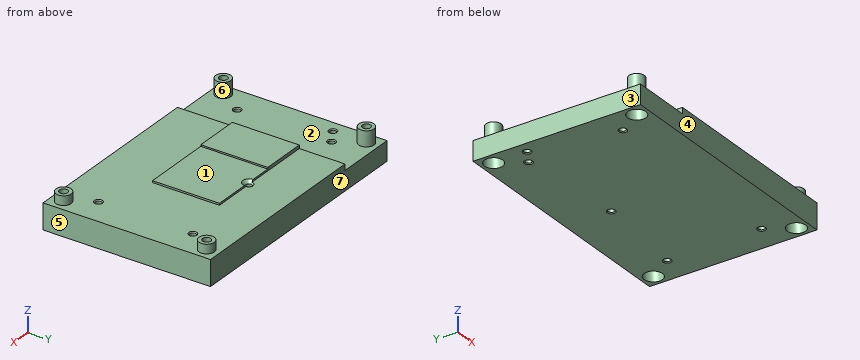
```python
from build123d import *

# Parameters (mm, degrees)
SKETCH1_W                               = 84
SKETCH1_H                               = 55
EXTRUDE1_DEPTH                          = 11.4
F_2_7_2_7_DIAMETER_HOLE1_D              = 2.7
SKETCH6_OUTSIDE_W                       = 106.21
SKETCH6_OUTSIDE_H                       = 77.21
SKETCH6_OUTSIDE_R                       = 2.5
EXTRUDE2_DEPTH                          = 3
SKETCH7_W                               = 15
SKETCH7_H                               = 22
EXTRUDE3_DEPTH                          = 1.1
SKETCH8_W                               = 26.471562954
SKETCH8_H                               = 62.575334395
SKETCH8_R                               = 2.5
EXTRUDE6_DEPTH                          = 2
SKETCH9_W                               = 23
SKETCH9_H                               = 22
EXTRUDE7_DEPTH                          = 0.6
M2_5X0_45_TAPPED_HOLE1_D                = 2.05
CBORE_FOR_M5_HEX_HEAD_BOLT1_D           = 2.7
CBORE_FOR_M5_HEX_HEAD_BOLT1_CBORE_D     = 6
CBORE_FOR_M5_HEX_HEAD_BOLT1_CBORE_DEPTH = 3.5
CHAMFER1_SIZE                           = 0.3


with BuildPart() as part:
    # Sketch1 → Extrude1 (new body)
    with BuildSketch(Plane.XY):
        Rectangle(SKETCH1_W, SKETCH1_H)
    extrude(amount=EXTRUDE1_DEPTH)

    # 2.7 _2.7_ Diameter Hole1 (through all)
    with Locations(Plane.XY.offset(11.4)):
        with Locations((-38, 23.5), (38, 23.5), (38, -23.5), (-38, -23.5)):
            Hole(F_2_7_2_7_DIAMETER_HOLE1_D / 2)

    # Sketch6 outside → Extrude2 (cut)
    with BuildSketch(Plane.XY.offset(11.4)):
        Rectangle(SKETCH6_OUTSIDE_W, SKETCH6_OUTSIDE_H)
        with Locations((-38, 23.5)):
            Circle(SKETCH6_OUTSIDE_R, mode=Mode.SUBTRACT)
        with Locations((-38, -23.5)):
            Circle(SKETCH6_OUTSIDE_R, mode=Mode.SUBTRACT)
        with Locations((38, 23.5)):
            Circle(SKETCH6_OUTSIDE_R, mode=Mode.SUBTRACT)
        with Locations((38, -23.5)):
            Circle(SKETCH6_OUTSIDE_R, mode=Mode.SUBTRACT)
    extrude(amount=-EXTRUDE2_DEPTH, mode=Mode.SUBTRACT)

    # Sketch7 → Extrude3 (add)
    with BuildSketch(Plane.XY.offset(8.4)):
        with Locations((-14.5, 1.5)):
            Rectangle(SKETCH7_W, SKETCH7_H)
    extrude(amount=EXTRUDE3_DEPTH)

    # Sketch8 → Extrude6 (cut)
    with BuildSketch(Plane.XY.offset(8.4)):
        with Locations((-35.235781477, -1.105270853)):
            Rectangle(SKETCH8_W, SKETCH8_H)
        with Locations((-38, -23.5)):
            Circle(SKETCH8_R, mode=Mode.SUBTRACT)
        with Locations((-38, 23.5)):
            Circle(SKETCH8_R, mode=Mode.SUBTRACT)
    extrude(amount=-EXTRUDE6_DEPTH, mode=Mode.SUBTRACT)

    # Sketch9 → Extrude7 (add)
    with BuildSketch(Plane.XY.offset(8.4)):
        with Locations((4.5, 1.5)):
            Rectangle(SKETCH9_W, SKETCH9_H)
    extrude(amount=EXTRUDE7_DEPTH)

    # M2.5x0.45 Tapped Hole1 (through all)
    with Locations(Plane.XY.offset(11.4)):
        with Locations((-33, 15.5), (33, 15.5), (33, -15.5), (-33, -15.5), (2, 12.5), (-38, 12.5)):
            Hole(M2_5X0_45_TAPPED_HOLE1_D / 2)

    # CBORE for M5 Hex Head Bolt1 (through all)
    with Locations(Plane(origin=(0, 0, 0), x_dir=(-1, 0, 0), z_dir=(0, 0, -1))):
        with Locations((-38, 23.5), (-38, -23.5), (38, 23.5), (38, -23.5)):
            CounterBoreHole(CBORE_FOR_M5_HEX_HEAD_BOLT1_D / 2, CBORE_FOR_M5_HEX_HEAD_BOLT1_CBORE_D / 2, CBORE_FOR_M5_HEX_HEAD_BOLT1_CBORE_DEPTH)

    # Chamfer1
    chamfer1_edges = [part.edges().sort_by_distance(p)[0] for p in [
        (-36.975, 12.5, 0),
        (-36.975, 12.5, 6.4),
        (3.025, 12.5, 0),
        (-31.975, -15.5, 0),
        (-31.975, -15.5, 6.4),
        (34.025, -15.5, 8.4),
        (34.025, -15.5, 0),
        (34.025, 15.5, 8.4),
        (34.025, 15.5, 0),
        (-31.975, 15.5, 0),
        (-31.975, 15.5, 6.4),
    ]]
    chamfer(chamfer1_edges, length=CHAMFER1_SIZE)

    # Sketch12 → Cut-Revolve1 (revolve, cut)
    with BuildSketch(Plane.ZY.offset(-2), mode=Mode.PRIVATE) as cut_revolve1_sk:
        Polygon((6.996424716, 12.489411428), (9.321943828, 14.81493054), (9.321943828, 12.489411428), align=None)
    revolve(cut_revolve1_sk.sketch.rotate(Axis((2, 12.489411428, 7.765521671), (0, 0, 1)), 270.302801858), axis=Axis((2, 12.489411428, 7.765521671), (0, 0, 1)), mode=Mode.SUBTRACT)  # turned: the seam where the file's is


solid = part.part
```
CAD build for the part. Positions are in the model's coordinates, mm. Face numbers are marked on the shaded views. A direction names the side the tool comes from. Round coordinates to 2 decimals unless told otherwise and drop trailing zeros. Write each loop counter-clockwise with the first axis right and the second up, starting at its lowest first coordinate (ties: lowest second). Pieces come first, ordered by that corner, then holes. Notation, with made-up numbers: (42.5, -10) - (63.5, -10) arc R12 ccw to (63.5, 5) - close; hole circle Ø9 at (53, -2.5). An arc over 180 degrees is marked (long way). Return JSON: item names as keys, results as strings. Group by question number.
Item 1: 3-axis set-ups, long thin cutter, end or side, ignore diameter. For the marked faces 1, 2 and 3: which of +Z, -Z, +X, -X, +Y, -Y reach the whole face in a straight line?
Item 2: Band-saw the part on A-A on x = 38. List the corners of the cut face in (y, z), plus the area to 3 significant figures.
Item 3: Band-saw the part on B-B on z = 2. State how many separate pieces and enclosed holes the cut face has, plus the area to 3 significant figures.
Item 4: Probe probe 1 along Y at (x, z) = (-38, 7.5); probe 2 along Y at (x, z) = (-33, 3.7) (3 decimals); probe 3 along Y at (x, z) = (-38, 3.45) (3 decimals). List the from-to ranges inside material, lowest first.
Item 5: Mould opens along Y. For the marked faces 4, 5, 6 and 7 say: +Y half, -Y half, draft (parallel to the pull), parting line (faces both ways), or undercut.
Item 6: Band-saw the part on D-D on x = -8. List the corners of the cut face in (y, z).
Item 7: Band-saw the part on C-C on y = -15.5. List the corners of the cut face in (x, z) (3 decimals), plus the area to 3 significant figures.
Item 8: Flat gauge pins, fed straight in: pin 1 Ø3.5 at (x, y) = (2, 12.5) entering from +Z; pin 2 Ø2.5 at (y, z) = (-5.5, 8) entering from -X; pin 3 Ø16 at (x, y) = (-28, -11.5) entering from +Z. Where does each tip first touch, or does it go through?
Resolved:
{
 "1": {"face 1": "+Z, +X, +Y, -Y", "face 2": "+Z", "face 3": "+Z, -Z, -X, +Y, -Y"},
 "2": {"outline": "(-27.5, 0) - (-26.5, 0) - (-26.5, 3.5) - (-24.85, 3.5) - (-24.85, 11.4) - (-26, 11.4) - (-26, 8.4) - (-27.5, 8.4) - close; (-22.15, 3.5) - (-20.5, 3.5) - (-20.5, 0) - (20.5, 0) - (20.5, 3.5) - (22.15, 3.5) - (22.15, 11.4) - (21, 11.4) - (21, 8.4) - (-21, 8.4) - (-21, 11.4) - (-22.15, 11.4) - close; (24.85, 3.5) - (26.5, 3.5) - (26.5, 0) - (27.5, 0) - (27.5, 8.4) - (26, 8.4) - (26, 11.4) - (24.85, 11.4) - close", "area": "407 mm²"},
 "3": {"separate pieces": "1", "enclosed holes": "10", "area": "4,490 mm²"},
 "4": {"probe 1": "y = -26 to -24.85, -22.15 to -21, 21 to 22.15, 24.85 to 26", "probe 2": "y = -27.5 to -16.525, -14.475 to 14.475, 16.525 to 27.5", "probe 3": "y = -27.5 to -26.5, -20.5 to 11.475, 13.525 to 20.5, 26.5 to 27.5"},
 "5": {"face 4": "-Y half", "face 5": "draft", "face 6": "undercut", "face 7": "+Y half"},
 "6": {"outline": "(-27.5, 0) - (27.5, 0) - (27.5, 8.4) - (12.5, 8.4) - (12.5, 9.5) - (-9.5, 9.5) - (-9.5, 8.4) - (-27.5, 8.4) - close"},
 "7": {"outline": "(-42, 0) - (-34.325, 0) - (-34.025, 0.3) - (-34.025, 6.1) - (-34.325, 6.4) - (-42, 6.4) - close; (-31.975, 0.3) - (-31.675, 0) - (31.675, 0) - (31.975, 0.3) - (31.975, 8.1) - (31.675, 8.4) - (-22, 8.4) - (-22, 6.4) - (-31.675, 6.4) - (-31.975, 6.1) - close; (34.025, 0.3) - (34.325, 0) - (42, 0) - (42, 8.4) - (34.325, 8.4) - (34.025, 8.1) - close", "area": "635 mm²"},
 "8": {"pin 1": "stops at z = 8.75", "pin 2": "stops at x = -22", "pin 3": "stops at z = 9.5"}
}
